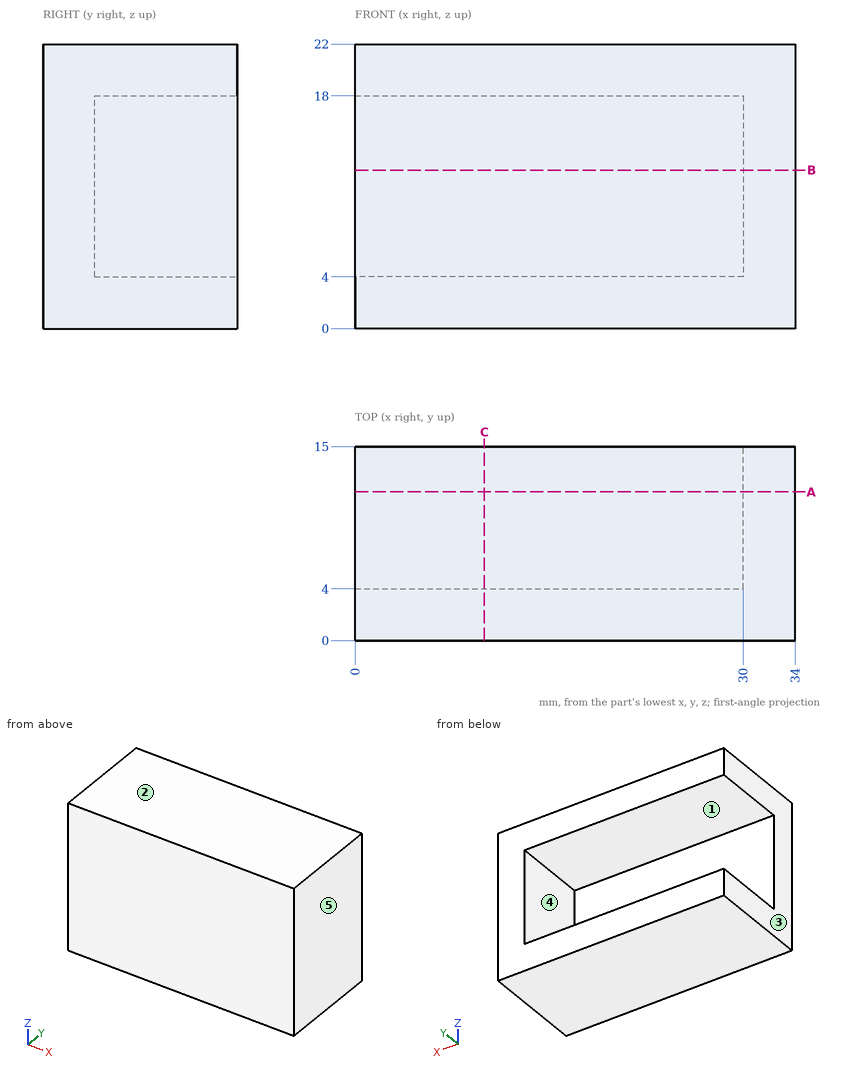
Geometry: see drawing. Coordinates: mm, zero at the bounding-box minimum. A direction names the side the tool comes from. Give positions to 0.01 mm unless a question says otherwise; leave off trailing zeros. Write each loop counter-clockwise with the first axis right and the second up, starting at its lowest first coordinate (ties: lowest second). Pieces come first, ordered by that corner, then holes. Notation, with made-up numbers: (62.5, -3) -> (119.5, -3) arc R22 ccw to (119.5, 13) -> close; hole circle Ø3 at (14, -40). An arc over 180 degrees is marked (long way). Use one line per item in the form item = value. Start each with the question number.
1) Section query B-B on z = 12.25. Return the cut outline in (x, y).
2) Section query A-A on y = 11.5. Return the cut outline in (x, z), then the cut area to 3 significant figures.
3) Set-up query: the marked faces 4 and 5. Return all of +Z, -Z, +X, -X, +Y, -Y with unobstructed straight access to the full face (end or side cutting, diameter ignored); none if empty.
4) Section query C-C on x = 10. Return the cut outline in (y, z), then the cut area to 3 significant figures.
5) Ray query, probe 1 along Z at (x, y) = (19.5, 11); probe 2 along Y at (x, z) = (3, 11.5); probe 3 along X at (y, z) = (4.75, 9.5). Return the intervals inside material, ascending. Write a range as from..to.
6) Draft query along Z for the marked faces 1, 2 and 3. Return one class per face: pulls with the +Z half, pulls with the -Z half, needs draft (parallel to the pull), parting line crosses it, or undercut.
7) Pin query (flat end, axial travel): pin 1 (11 mm diameter, centred on x = 19.5, z = 12, fed in from +Y); pin 2 (8 mm diameter, centred on x = 29, z = 5.5, fed in from -Y); pin 3 (5 mm diameter, centred on y = 10, z = 11.5, fed in from -X). Return the tip coordinate at first contact, or that it passes through.
Outcome:
q1.outline = (0, 0) -> (34, 0) -> (34, 15) -> (30, 15) -> (30, 4) -> (0, 4) -> close
q2.outline = (0, 0) -> (34, 0) -> (34, 22) -> (0, 22) -> (0, 18) -> (30, 18) -> (30, 4) -> (0, 4) -> close
q2.area = 328 mm^2
q3.face_4 = -X, +Y
q3.face_5 = +Z, -Z, +X, +Y, -Y
q4.outline = (0, 0) -> (15, 0) -> (15, 4) -> (4, 4) -> (4, 18) -> (15, 18) -> (15, 22) -> (0, 22) -> close
q4.area = 176 mm^2
q5.probe_1 = 0..4, 18..22
q5.probe_2 = 0..4
q5.probe_3 = 30..34
q6.face_1 = undercut
q6.face_2 = pulls with the +Z half
q6.face_3 = needs draft
q7.pin_1 = 4
q7.pin_2 = 0
q7.pin_3 = 30
